```python
from build123d import *

# Parameters (mm, degrees)
F1_DEPTH = 25.5
F2_W     = 26.5
F2_H     = 2
F3_DEPTH = 18.001
F4_DEPTH = 13.848382
F6_DEPTH = 3.2


with BuildPart() as f1:
    # F0 (on Top) → F1 (new body)
    with BuildSketch(Plane.XY):
        with BuildLine():
            Line((11.5, 0), (11.5, -13.847382))
            ThreePointArc((11.5, -13.847382), (0, 18), (-11.5, -13.847382))
            Line((-11.5, -13.847382), (-11.5, 0))
            ThreePointArc((-11.5, 0), (0, 11.5), (11.5, 0))
        make_face()
    extrude(amount=F1_DEPTH)

    # F2 (on Front) → F3 (cut, through all)
    with BuildSketch(Plane.XZ):
        Polygon((-13.25, 23.5), (-14.25, 23.5), (-14.25, 17.5), (14.25, 17.5), (14.25, 23.5), (13.25, 23.5), align=None)
        with Locations((0, 24.5)):
            Rectangle(F2_W, F2_H)
    extrude(amount=-F3_DEPTH, mode=Mode.SUBTRACT)

    # F2 (on Front) → F4 (cut, through all)
    with BuildSketch(Plane.XZ):
        Polygon((-13.25, 23.5), (-14.25, 23.5), (-14.25, 17.5), (14.25, 17.5), (14.25, 23.5), (13.25, 23.5), align=None)
        with Locations((0, 24.5)):
            Rectangle(F2_W, F2_H)
    extrude(amount=F4_DEPTH, mode=Mode.SUBTRACT)

    # F5 (on face) → F6 (cut)
    with BuildSketch(Plane(origin=(0, 0, 0), x_dir=(1, 0, 0), z_dir=(0, 0, -1))):
        with BuildLine():
            ThreePointArc((-11.5, 13.847382), (-15.961029, 8.32139), (-17.937391, 1.5))
            Line((-17.937391, 1.5), (-11.5, 1.5))
            Line((-11.5, 1.5), (-11.5, 13.847382))
        make_face()
        with BuildLine():
            ThreePointArc((-17.937391, -1.5), (-12.727922, -12.727922), (-1.5, -17.937391))
            Line((-1.5, -17.937391), (-1.5, -11.401754))
            ThreePointArc((-1.5, -11.401754), (-8.131728, -8.131728), (-11.401754, -1.5))
            Line((-11.401754, -1.5), (-17.937391, -1.5))
        make_face()
        with BuildLine():
            Line((1.5, -11.401754), (1.5, -17.937391))
            ThreePointArc((1.5, -17.937391), (12.727922, -12.727922), (17.937391, -1.5))
            Line((17.937391, -1.5), (11.401754, -1.5))
            ThreePointArc((11.401754, -1.5), (8.131728, -8.131728), (1.5, -11.401754))
        make_face()
        with BuildLine():
            Line((11.5, 1.5), (17.937391, 1.5))
            ThreePointArc((17.937391, 1.5), (15.961029, 8.32139), (11.5, 13.847382))
            Line((11.5, 13.847382), (11.5, 1.5))
        make_face()
    extrude(amount=-F6_DEPTH, mode=Mode.SUBTRACT)


solid = f1.part
```
Source: CAD feature listing. Evaluate the final solid. Frame: model axes, mm. A direction names the side the tool comes from. Round coordinates to 2 decimals unless told otherwise and drop trailing zeros. Loops run counter-clockwise (first coordinate to the right, second up) from the corner with the lowest first, then second, coordinate; pieces in that order, holes last. Notation, with made-up numbers: (65.25, 22.5) - (119.25, 22.5) arc R32 ccw to (119.25, 59.5) - close; hole circle Ø6 at (6, 9.25). An arc over 180 degrees is marked (long way). Use CSV: the item, a comma, the result in double quotes.
Q1. Section query D-D, the plane y = 2. Output: boundary loops of the cut face in (x, z), then the cut area to 3 significant figures.
Reported:
outline,"(-17.89, 3.2) - (-11.32, 3.2) - (-11.32, 17.5) - (-14.25, 17.5) - (-14.25, 23.5) - (-13.25, 23.5) - (-13.25, 25.5) - (-17.89, 25.5) - close; (11.32, 3.2) - (17.89, 3.2) - (17.89, 25.5) - (13.25, 25.5) - (13.25, 23.5) - (14.25, 23.5) - (14.25, 17.5) - (11.32, 17.5) - close"
area,"250 mm^2"
Q2. Reachability of faces 4 (the flat face through (15, 1.5, 2)), 5 (the flat face through (14.25, 0, 20)), 6 (the flat face through (-13.25, 0, 24)), 7 (the flat face through (15, -1.5, 2)), 8 (the flat face through (-11.5, -7, 11)) from +Z, -Z, +X, -X, +Y, -Y: full face, straight path, thin tool, end or side. Return the list, or none.
Reported:
face 4,"-Z, +X, -X, +Y"
face 5,"+Y, -Y"
face 6,"+Z, +Y, -Y"
face 7,"-Z, +X, -X, -Y"
face 8,"+Z, -Z, -Y"
Q3. Ray query, line 1 along Z through (x, y) = (13.5, -4); line 2 along Z through (x, y) = (-8, 12.5); line 3 along X through (y, z) = (6, 6). Return the intervals inside material, ascending.
Reported:
line 1,"3.2 to 17.5, 23.5 to 25.5"
line 2,"3.2 to 17.5"
line 3,"-16.97 to -9.81, 9.81 to 16.97"
Q4. Section query A-A, the plane y = 10. Output: boundary loops of the cut face in (x, z).
Reported:
outline,"(-14.97, 3.2) - (-5.68, 3.2) - (-5.68, 17.5) - (-14.25, 17.5) - (-14.25, 23.5) - (-13.25, 23.5) - (-13.25, 25.5) - (-14.97, 25.5) - close; (5.68, 3.2) - (14.97, 3.2) - (14.97, 25.5) - (13.25, 25.5) - (13.25, 23.5) - (14.25, 23.5) - (14.25, 17.5) - (5.68, 17.5) - close"
Q5. Section query B-B, the plane z = 18.25. Output: boundary loops of the cut face in (x, y), then the cut area to 3 significant figures.
Reported:
outline,"(-14.25, -11) - (-14.25, 11) arc R18 ccw to start; (14.25, -11) arc R18 ccw to (14.25, 11) - close"
area,"112 mm^2"
Q6. Pin query (flat end, axial travel): pin 1 Ø1.5 at (y, z) = (-5, 20.5) entering from -X; pin 2 Ø5 at (x, z) = (3.5, 5) entering from +Y; pin 3 Ø0.6 at (y, z) = (4, 24) entering from -X. Return the tip coordinate at first contact, or that it passes through.
Reported:
pin 1,"x = -17.49"
pin 2,"y = 17.97"
pin 3,"x = -17.62"
Q7. Mould query, pull axis X, two halves, no side actions, for faces 1 (the flat face through (1.5, 15, 2)), 2 (the flat face through (14, -6, 3.2)), 3 (the flat face through (-14.25, 0, 21)). Classes: pulls with the +X half, pulls with the -X half, needs draft (parallel to the pull), parting line crosses it, or undercut.
Reported:
face 1,"pulls with the +X half"
face 2,"needs draft"
face 3,"undercut"
Q8. Section query C-C, the plane x = 0. Output: boundary loops of the cut face in (y, z).
Reported:
outline,"(11.5, 0) - (18, 0) - (18, 17.5) - (11.5, 17.5) - close"
